The drawing under review shows one solid part. Ordinate dimensions are in mm from its lowest x, y, z. Give positions to 0.01 mm unless a question says otherwise; leave off trailing zeros. Loops run counter-clockwise (first coordinate to the right, second up) from the corner with the lowest first, then second, coordinate; pieces in that order, holes last. Notation, with made-up numbers: (11.25, 39) - (40.25, 39) arc R21 cw to (40.25, 60) - close; hole circle Ø7 at (-3, -21.5). An arc over 180 degrees is marked (long way). One line per item, written item: value. Start each with the question number.
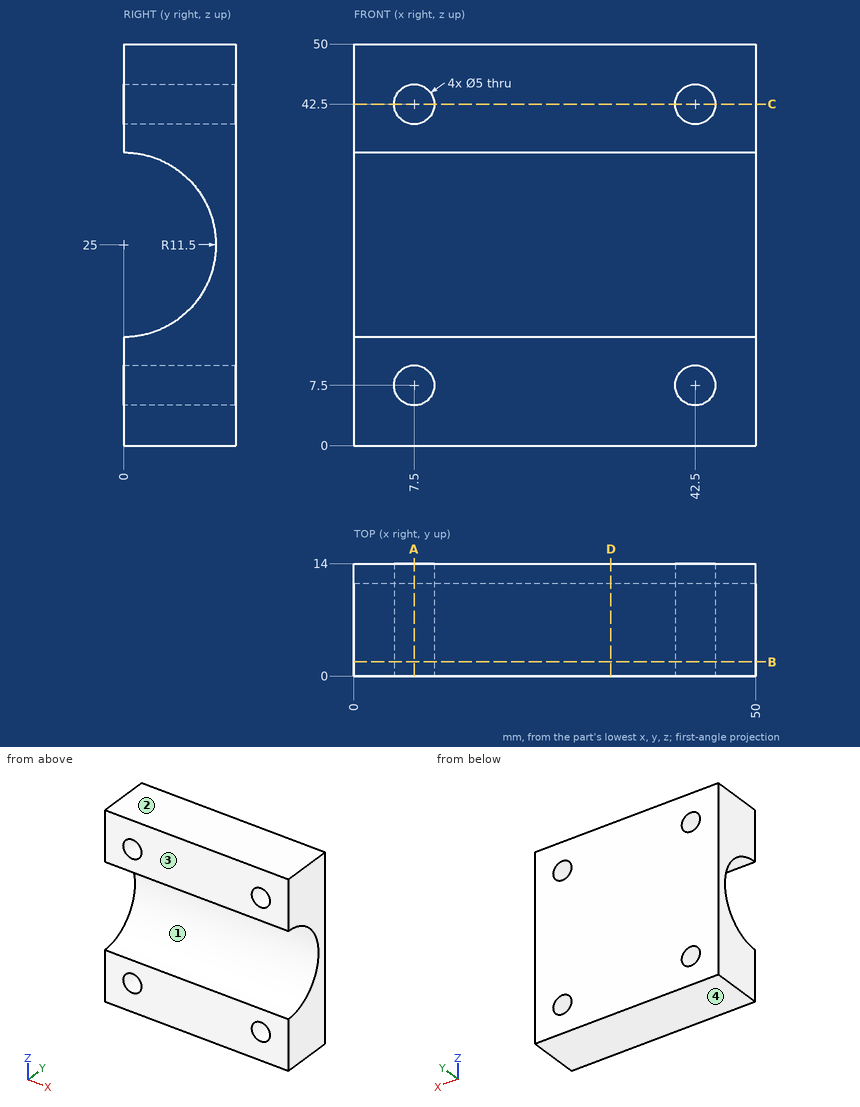
(1) Take a section at D-D on x = 32. State the section outline as (y, z) points.
(2) Take a section at A-A on x = 7.5. State the section outline as (y, z) points.
(3) Take a section at C-C on z = 42.5. State the section outline as (x, y) points, and give its area (3 significant figures).
(4) Take a section at B-B on y = 1.75. State the section outline as (x, z) points.
(5) Draft analysis for pull direction Z (two halves, no side actions). For the marked faces 1, 2, 3 and 4, state which applies: pulls with the +Z half, pulls with the -Z half, needs draft (parallel to the pull), parting line crosses it, or undercut.
(6) To check wall thickness, follow L1, parallel to X at y = 6.5, z = 7.5; L2, parallel to Z at x = 44.5, y = 12; L3, parallel to Z at x = 8.5, y = 6.5. State the ranges of each line that lie inside material, in increasing order. Write a range as from..to.
Here are the results:
1. outline: (0, 0) - (14, 0) - (14, 50) - (0, 50) - (0, 36.5) arc R11.5 cw to (0, 13.5) - close
2. outline: (0, 0) - (14, 0) - (14, 5) - (0, 5) - close; (0, 10) - (14, 10) - (14, 40) - (0, 40) - (0, 36.5) arc R11.5 cw to (0, 13.5) - close; (0, 45) - (14, 45) - (14, 50) - (0, 50) - close
3. outline: (0, 0) - (5, 0) - (5, 14) - (0, 14) - close; (10, 0) - (40, 0) - (40, 14) - (10, 14) - close; (45, 0) - (50, 0) - (50, 14) - (45, 14) - close
3. area: 560 mm²
4. outline: (0, 0) - (50, 0) - (50, 13.63) - (0, 13.63) - close; (0, 36.37) - (50, 36.37) - (50, 50) - (0, 50) - close; hole circle Ø5 at (7.5, 7.5); hole circle Ø5 at (7.5, 42.5); hole circle Ø5 at (42.5, 7.5); hole circle Ø5 at (42.5, 42.5)
5. face 1: undercut
5. face 2: pulls with the +Z half
5. face 3: needs draft
5. face 4: pulls with the -Z half
6. L1: 0..5, 10..40, 45..50
6. L2: 0..6, 9..41, 44..50
6. L3: 0..5.21, 9.79..15.51, 34.49..40.21, 44.79..50
